from build123d import *

# Parameters (mm, degrees)
BOSS_EXTRUDE1_DEPTH = 2.8


with BuildPart() as part:
    # Sketch1 → Boss-Extrude1 (new body)
    with BuildSketch(Plane.XY):
        Polygon((40.979118187, 112.870740647), (-14.14721608, 112.870740647), (-75.508978364, 51.508978364), (-3, -21), (31.617964081, -21), align=None)
        Polygon((-2.943243377, -1), (2.943243377, -1), (10.193422936, 102.682398168), (7.5, 102.870740647), (7.15036594, 97.870740647), (-7.15036594, 97.870740647), (-7.5, 102.870740647), (-10.193422936, 102.682398168), align=None, mode=Mode.SUBTRACT)
    extrude(amount=BOSS_EXTRUDE1_DEPTH)


solid = part.part
The listing builds one solid part. Answer for the finished solid, in the listing's coordinates (mm). A direction names the side the tool comes from. Coordinates: 2 decimals unless noted, no trailing zeros. Order: outer loops, then holes, each group sorted by start corner. A loop starts at its lowest first (then second) coordinate and runs counter-clockwise, first axis right, second up. Notation, with made-up numbers: M 39.5,53.25 L 88.5,53.25 A16 ccw 88.5,61.25 Z; hole C 86,68 d4. An arc over 180 degrees is marked long. Use CSV: the item, a comma, the result in double quotes.
Q1. Determine the mould class of faces 1 (the flat face through (8.866, 102.775, 1.38)), 2 (the flat face through (-8.828, 102.778, 1.38)), 3 (the flat face through (-44.4, 82.62, 1.38)), 4 (the flat face through (8, 47, 0)) for opening direction X: pulls with the +X half, pulls with the -X half, needs draft (parallel to the pull), parting line crosses it, or undercut.
Here are the results:
face 1,"undercut"
face 2,"undercut"
face 3,"pulls with the -X half"
face 4,"needs draft"
Q2. Section B-B (y = 12) is taken. Determine the outline of the cut face in (x, z).
Here are the results:
outline,"M -36,0 L -3.85,0 L -3.85,2.8 L -36,2.8 Z; M 3.85,0 L 33.93,0 L 33.93,2.8 L 3.85,2.8 Z"
Q3. Section A-A (z = 0.95) is taken. Determine the outline of the cut face in (x, y).
Here are the results:
outline,"M -75.51,51.51 L -3,-21 L 31.62,-21 L 40.98,112.87 L -14.15,112.87 Z; hole M -10.19,102.68 L -2.94,-1 L 2.94,-1 L 10.19,102.68 L 7.5,102.87 L 7.15,97.87 L -7.15,97.87 L -7.5,102.87 Z"
Q4. A tool of negligible diameter and unlimited length cuts with its end or side. For faces 5 (the flat face through (0, -1, 1)), 6 (the flat face through (14, -21, 1)), from which of +Z, -Z, +X, -X, +Y, -Y can it reach the whole face along a straight path? Write none if from no direction.
Here are the results:
face 5,"+Z, -Z"
face 6,"+Z, -Z, +X, -X, -Y"
Q5. Straight lines are drawn through the part: L1, parallel to X at y = 102, z = 1.35; L2, parallel to X at y = 58.5, z = 1.55; L3, parallel to X at y = 53, z = 1.6. For each, find the intervals that lie inside material, in ascending order.
Here are the results:
L1,"-25.02 to -10.15, -7.44 to 7.44, 10.15 to 40.22"
L2,"-68.52 to -7.1, 7.1 to 37.18"
L3,"-74.02 to -6.72, 6.72 to 36.79"
Q6. Section C-C (y = 53) is taken. Determine the outline of the cut face in (x, z), then the cut area to 3 significant figures.
Here are the results:
outline,"M -74.02,0 L -6.72,0 L -6.72,2.8 L -74.02,2.8 Z; M 6.72,0 L 36.79,0 L 36.79,2.8 L 6.72,2.8 Z"
area,"273 mm2"
Q7. Given pin 1 Ø1 at (x, z) = (-63, 2) entering from +Y; pin 2 Ø6 at (x, y) = (2.5, 92.5) entering from -Z (1 decimal), each flat-ended and moving along its own axis, determine where each tip first touches the part or whether it passes through.
Here are the results:
pin 1,"y = 64.52"
pin 2,"through"
Q8. Section D-D (x = -63) is taken. Determine the outline of the cut face in (y, z), then the cut area to 3 significant figures.
Here are the results:
outline,"M 39,0 L 64.02,0 L 64.02,2.8 L 39,2.8 Z"
area,"70.1 mm2"
